Work out the finished part from the listing and answer in its coordinate system (mm). Coordinates: 2 decimals unless noted, no trailing zeros. Order: outer loops, then holes, each group sorted by start corner. A loop starts at its lowest first (then second) coordinate and runs counter-clockwise, first axis right, second up. Notation, with made-up numbers: M 61.25,30 L 72.25,30 A37 ccw 72.25,66 Z; hole C 62,65 d8. An arc over 180 degrees is marked long. Use a Markdown table: item, result.
from build123d import *

# Parameters (mm, degrees)
SKETCH1_W                       = 2
SKETCH1_H                       = 6.4
BOSS_EXTRUDE1_DEPTH             = 36.4
CUT_EXTRUDE8_DEPTH              = 37.595081637
CUT_EXTRUDE8_DEPTH_BACK         = 37.595081637
SKETCH15_W                      = 2
SKETCH15_H                      = 0.75
CUT_EXTRUDE5_DEPTH              = 72.8
M2X0_4_TAPPED_HOLE1_D           = 1.6
M2X0_4_TAPPED_HOLE1_DEPTH       = 3.6
M2X0_4_TAPPED_HOLE1_TIP         = 0.480688495
CUT_EXTRUDE9_DEPTH              = 37.595081637
CUT_EXTRUDE9_DEPTH_BACK         = 37.595081637
BOSS_EXTRUDE8_REACH             = 38.595
BOSS_EXTRUDE8_DIRECTION_2_REACH = 38.595
FILLET7_R                       = 1


with BuildPart() as part:
    # Sketch1 → Boss-Extrude1 (new, symmetric)
    with BuildSketch(Plane(origin=(0, 0, 0), x_dir=(0, 0, -1), z_dir=(1, 0, 0))):
        with Locations((-1, 0)):
            Rectangle(SKETCH1_W, SKETCH1_H)
    extrude(amount=BOSS_EXTRUDE1_DEPTH, both=True)

    # Sketch15 → Cut-Extrude8 (cut, two sides: drawn at the far end of the back side and taken through both)
    with BuildSketch(Plane(origin=(0, 0, 0), x_dir=(0, 0, -1), z_dir=(1, 0, 0)).offset(-CUT_EXTRUDE8_DEPTH_BACK)):
        with Locations((-1, 2.825)):
            Rectangle(SKETCH15_W, SKETCH15_H)
    extrude(amount=CUT_EXTRUDE8_DEPTH + CUT_EXTRUDE8_DEPTH_BACK, mode=Mode.SUBTRACT)

    # Sketch5 → Cut-Extrude5 (cut)
    with BuildSketch(Plane.ZY.offset(36.4)):
        Polygon((0, -3.2), (0.5, -3.2), (0, -2.7), align=None)
    extrude(amount=-CUT_EXTRUDE5_DEPTH, mode=Mode.SUBTRACT)

    # M2x0.4 Tapped Hole1
    with Locations(Plane.XY.offset(2)):
        with Locations((-22, -0.2), (22, -0.2), (0, -0.2)):
            Hole(M2X0_4_TAPPED_HOLE1_D / 2, depth=M2X0_4_TAPPED_HOLE1_DEPTH)
            with Locations((0, 0, -(M2X0_4_TAPPED_HOLE1_DEPTH + M2X0_4_TAPPED_HOLE1_TIP / 2))):  # 118° drill point
                Cone(0, M2X0_4_TAPPED_HOLE1_D / 2, M2X0_4_TAPPED_HOLE1_TIP, mode=Mode.SUBTRACT)

    # Sketch16 → Cut-Extrude9 (cut, two sides: drawn at the far end of the back side and taken through both)
    with BuildSketch(Plane(origin=(0, 0, 0), x_dir=(0, 0, -1), z_dir=(1, 0, 0)).offset(-CUT_EXTRUDE9_DEPTH_BACK)):
        Polygon((0, 3.2), (-2, 3.2), (-2, 1.2), align=None)
    extrude(amount=CUT_EXTRUDE9_DEPTH + CUT_EXTRUDE9_DEPTH_BACK, mode=Mode.SUBTRACT)

    # Boss-Extrude8: up to this face of the body (flat: up to its plane)
    boss_extrude8_end = Plane(part.part.faces().sort_by_distance((36.4, -0.524052916, 0.966175586))[0])
    # Sketch17 → Boss-Extrude8 (add, up to the picked face)
    with BuildSketch(Plane(origin=(0, 0, 0), x_dir=(0, 0, -1), z_dir=(1, 0, 0)), mode=Mode.PRIVATE) as boss_extrude8_sk1:
        Polygon((0, 2.45), (1, 2.45), (1, -1.7), (0, -2.7), align=None)
    boss_extrude8_tool1 = split(extrude(boss_extrude8_sk1.sketch, amount=BOSS_EXTRUDE8_REACH, mode=Mode.PRIVATE), bisect_by=boss_extrude8_end, keep=Keep.BOTH, mode=Mode.PRIVATE)
    add(boss_extrude8_tool1.solids().sort_by(Axis((0, 0.116039, -0.482079), (1, 0, 0)))[0])

    # Boss-Extrude8 direction 2: up to this face of the body (flat: up to its plane)
    boss_extrude8_direction_2_end = Plane(part.part.faces().sort_by_distance((-36.4, -0.524052916, 0.966175586))[0])
    # Sketch17 → Boss-Extrude8 direction 2 (add, up to the picked face)
    with BuildSketch(Plane(origin=(0, 0, 0), x_dir=(0, 0, -1), z_dir=(1, 0, 0)), mode=Mode.PRIVATE) as boss_extrude8_direction_2_sk1:
        Polygon((0, 2.45), (1, 2.45), (1, -1.7), (0, -2.7), align=None)
    boss_extrude8_direction_2_tool1 = split(extrude(boss_extrude8_direction_2_sk1.sketch, amount=-BOSS_EXTRUDE8_DIRECTION_2_REACH, mode=Mode.PRIVATE), bisect_by=boss_extrude8_direction_2_end, keep=Keep.BOTH, mode=Mode.PRIVATE)
    add(boss_extrude8_direction_2_tool1.solids().sort_by(Axis((0, 0.116039, -0.482079), (-1, 0, 0)))[0])

    # Fillet7
    fillet7_edges = [part.edges().sort_by_distance(p)[0] for p in [
        (0, -1.7, -1),
    ]]
    fillet(fillet7_edges, radius=FILLET7_R)


solid = part.part
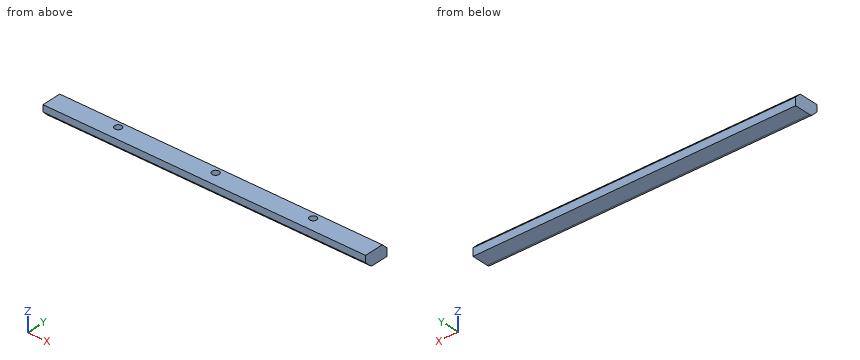
(1) Straight lines are drawn through the part: L1, parallel to X at y = -0.15, z = 1.05; L2, parallel to Y at x = 0, z = 0.6; L3, parallel to Y at x = -22, z = 1. For each, find the intervals that lie inside material, in ascending order.
Conclusion:
| item | result |
|---|---|
| L1 | -36.4 to -22.8, -21.2 to -0.8, 0.8 to 21.2, 22.8 to 36.4 |
| L2 | -3.2 to -1, 0.6 to 2.45 |
| L3 | -3.2 to -1, 0.6 to 2.2 |
(2) A cutting plane is placed at A-A (x = -22). Determine the outline of the cut face in (y, z), then the cut area to 3 significant figures.
Conclusion:
| item | result |
|---|---|
| outline | M -3.2,0.5 L -1.99,-0.71 A1 ccw -1.29,-1 L 2.45,-1 L 2.45,0.75 L 1.2,2 L 0.6,2 L 0.6,0 L -1,0 L -1,2 L -3.2,2 Z |
| area | 11.8 mm2 |
(3) Given P1, Ø0.5, axis at x = 0, y = 0, coming from the +Z side, flat-ended and moving along its own axis, determine where the tip first touches the part or whether it passes through.
Conclusion:
| item | result |
|---|---|
| P1 | z = 0 |
(4) A cutting plane is placed at B-B (x = -5). Determine the outline of the cut face in (y, z), then the cut area to 3 significant figures.
Conclusion:
| item | result |
|---|---|
| outline | M -3.2,0.5 L -1.99,-0.71 A1 ccw -1.29,-1 L 2.45,-1 L 2.45,0.75 L 1.2,2 L -3.2,2 Z |
| area | 15.0 mm2 |
